The figure shows three views and two pictorial views of one solid part (mm, origin at its lowest corner). Answer the questions. A direction names the side the tool comes from. Coordinates: 2 decimals unless noted, no trailing zeros. Order: outer loops, then holes, each group sorted by start corner. A loop starts at its lowest first (then second) coordinate and runs counter-clockwise, first axis right, second up. Notation, with made-up numbers: (-19.5, -14.5) - (37.5, -14.5) arc R3 ccw to (37.5, -10.5) - close; hole circle Ø1 at (-16.5, -11.75). An arc over 180 degrees is marked (long way). Use one line per item in the form item = value.
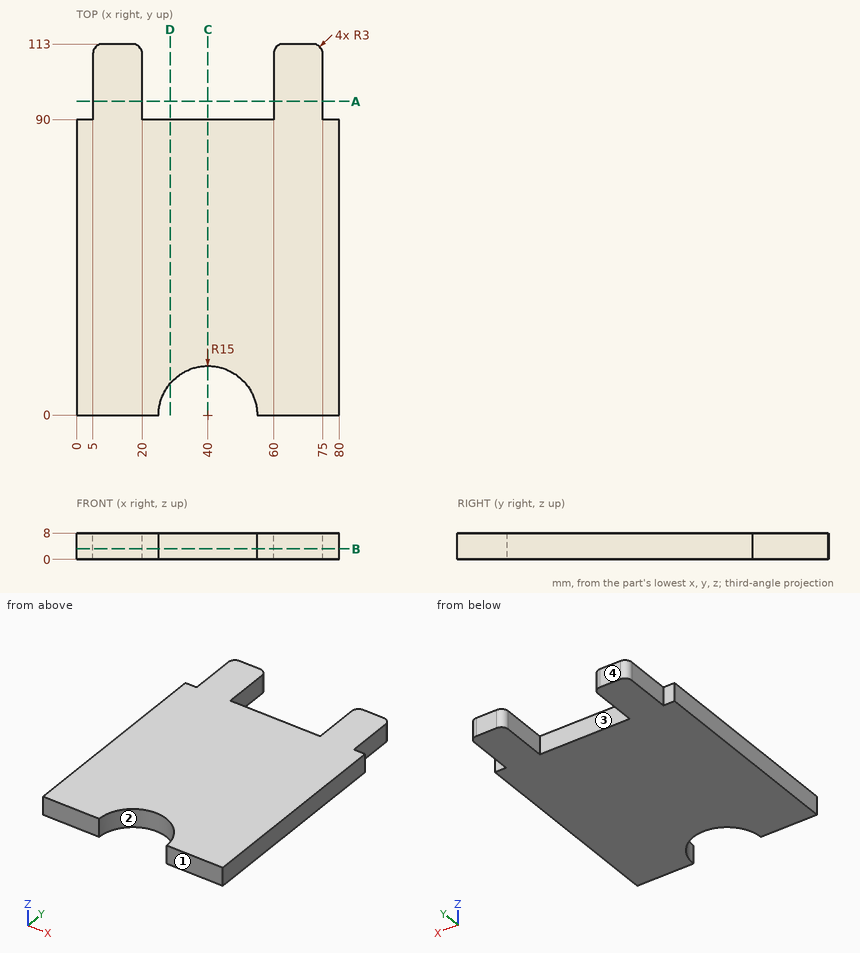
(1) The mould has two halves that part along X. Classify the marked faces 1 and 2: +X half, -X half, draft (parallel to the pull), parting line (faces both ways), or undercut.
Answer list:
face_1 = draft
face_2 = undercut
(2) Section C-C, the plane x = 40 is taken. Write down the section's boundary in (y, z).
Answer list:
outline = (15, 0) - (90, 0) - (90, 8) - (15, 8) - close
(3) Given pin 1 Ø4 at (y, z) = (93.5, 6.5) entering from -X; pin 2 Ø4 at (y, z) = (104, 6) entering from +X; pin 3 Ø2.5 at (x, z) = (3, 3.5) entering from +Y, each flat-ended and moving along its own axis, determine where each tip first touches the part or whether it passes through.
Answer list:
pin_1 = 5
pin_2 = 75
pin_3 = 90
(4) Section A-A, the plane y = 95.5 is taken. Write down the section's boundary in (x, z), then the cut area to 3 significant figures.
Answer list:
outline = (5, 0) - (20, 0) - (20, 8) - (5, 8) - close; (60, 0) - (75, 0) - (75, 8) - (60, 8) - close
area = 240 mm2
(5) Straight lines are drawn through the part: L1, parallel to X at y = 96, z = 2.25; L2, parallel to X at y = 10.5, z = 2.25; L3, parallel to Y at x = 62, z = 5.5. For each, find the intervals that lie inside material, in ascending order.
Answer list:
L1 = 5 to 20, 60 to 75
L2 = 0 to 29.29, 50.71 to 80
L3 = 0 to 112.83
(6) Which of the six approach directions +Z, -Z, +X, -X, +Y, -Y give full straight-line access (tool end or side, diameter ignored) to the marked faces 3 and 4?
Answer list:
face_3 = +Z, -Z, +Y
face_4 = +Z, -Z, +X, -X, +Y
(7) Section B-B, the plane z = 3.25 is taken. Write down the section's boundary in (x, y).
Answer list:
outline = (0, 0) - (25, 0) arc R15 cw to (55, 0) - (80, 0) - (80, 90) - (75, 90) - (75, 110) arc R3 ccw to (72, 113) - (63, 113) arc R3 ccw to (60, 110) - (60, 90) - (20, 90) - (20, 110) arc R3 ccw to (17, 113) - (8, 113) arc R3 ccw to (5, 110) - (5, 90) - (0, 90) - close
(8) Section D-D, the plane x = 28.5 is taken. Write down the section's boundary in (y, z).
Answer list:
outline = (9.63, 0) - (90, 0) - (90, 8) - (9.63, 8) - close
